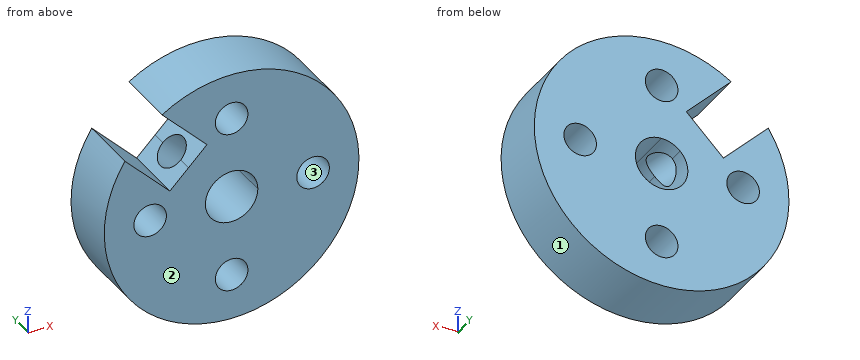
```python
from build123d import *

# Parameters (mm, degrees)
SKETCH_1_R          = 12.5
EXTRUDE_1_DEPTH     = 6
SKETCH_4_R          = 1.6
CUT_EXTRUDE_2_DEPTH = 30
CUT_EXTRUDE_3_DEPTH = 30
SKETCH_6_R          = 1.6
CUT_EXTRUDE_4_DEPTH = 6


with BuildPart() as part:
    # 草图1 → 凸台-拉伸1 (new body)
    with BuildSketch(Plane(origin=(0, 0, 0), x_dir=(1, 0, 0), z_dir=(0, 1, 0))):
        with Locations(Location((0, 0, 0), (0, 0, 270))):
            Circle(SKETCH_1_R)
    extrude(amount=EXTRUDE_1_DEPTH)

    # 草图4 → 切除-拉伸2 (cut)
    with BuildSketch(Plane(origin=(0, 0, 0), x_dir=(1, 0, 0), z_dir=(0, 1, 0))):
        with Locations(Location((0, 8, 0), (0, 0, 270))):
            Circle(SKETCH_4_R)
        with Locations(Location((8, 0, 0), (0, 0, 270))):
            Circle(SKETCH_4_R)
        with Locations(Location((0, -8, 0), (0, 0, 270))):
            Circle(SKETCH_4_R)
        with Locations(Location((-8, 0, 0), (0, 0, 270))):
            Circle(SKETCH_4_R)
    extrude(amount=CUT_EXTRUDE_2_DEPTH, mode=Mode.SUBTRACT)

    # 草图5 → 切除-拉伸3 (cut)
    with BuildSketch(Plane.XZ):
        with BuildLine():
            Line((-4.242640687, 4.242640687), (-8.838834765, 8.838834765))
            ThreePointArc((-8.838834765, 8.838834765), (-9.706634329, 7.875992001), (-10.470059323, 6.8284594))
            Line((-10.470059323, 6.8284594), (-6.063440649, 2.421840726))
            Line((-6.063440649, 2.421840726), (-4.242640687, 4.242640687))
        make_face()
        with BuildLine():
            ThreePointArc((-6.8284594, 10.470059323), (-7.875992001, 9.706634329), (-8.838834765, 8.838834765))
            Line((-8.838834765, 8.838834765), (-4.242640687, 4.242640687))
            Line((-4.242640687, 4.242640687), (-2.421840726, 6.063440649))
            Line((-2.421840726, 6.063440649), (-6.8284594, 10.470059323))
        make_face()
        with BuildLine():
            ThreePointArc((0, 2.575), (-0.985409838, 2.378989796), (-1.820799962, 1.820799962))
            Line((-1.820799962, 1.820799962), (0, 0))
            Line((0, 0), (0, 2.575))
        make_face()
        with BuildLine():
            Line((0, 0), (-1.820799962, 1.820799962))
            ThreePointArc((-1.820799962, 1.820799962), (-0.985409838, -2.378989796), (2.575, 0))
            ThreePointArc((2.575, 0), (1.820799962, 1.820799962), (0, 2.575))
            Line((0, 2.575), (0, 0))
        make_face()
    extrude(amount=-CUT_EXTRUDE_3_DEPTH, mode=Mode.SUBTRACT)

    # 草图6 → 切除-拉伸4 (cut)
    with BuildSketch(Plane(origin=(-4.242640687, 0, 4.242640687), x_dir=(0.7071067811865509, 0, 0.7071067811865442), z_dir=(-0.7071067811865442, 0, 0.7071067811865509))):
        with Locations((0, 3)):
            Circle(SKETCH_6_R)
    extrude(amount=-CUT_EXTRUDE_4_DEPTH, mode=Mode.SUBTRACT)


solid = part.part
```
Verification items for the finished model (mm, model axes). Face numbers are marked on the shaded views. Coordinates: 2 decimals unless noted, no trailing zeros. Loops run counter-clockwise (first coordinate to the right, second up) from the corner with the lowest first, then second, coordinate; pieces in that order, holes last. Notation, with made-up numbers: (83.5, 22.5) -> (119.5, 22.5) arc R20 ccw to (119.5, 33.5) -> close; hole circle Ø2 at (-10, -4.75). An arc over 180 degrees is marked (long way). Put each result on its own line as item: value.
1. Mould release check, pull along Z, two halves, no side actions. Record for the marked faces 1, 2 and 3: pulls with the +Z half, pulls with the -Z half, needs draft (parallel to the pull), parting line crosses it, or undercut.
Result set:
face 1: parting line crosses it
face 2: needs draft
face 3: undercut
2. Section check C-C, the plane y = 5.25. Record the boundary of the cut face in (x, z) (3 decimals).
Result set:
outline: (-10.47, 6.828) arc R12.5 ccw (long way) to (-6.828, 10.47) -> (-2.422, 6.063) -> (-6.063, 2.422) -> close; hole circle Ø3.2 at (-8, 0); hole circle Ø5.15 at (0, 0); hole circle Ø3.2 at (0, -8); hole circle Ø3.2 at (0, 8); hole circle Ø3.2 at (8, 0)
3. Gauge pin test, flat ends, axial feed: P1, Ø3, axis at x = 8, z = 0, coming from the +Y side; P2, Ø1.5, axis at y = 2, z = 3.5, coming from the +X side. Record the tip position at first contact, or that the pin passes through.
Result set:
P1: passes through
P2: stops at x = 12.19
4. Thickness scan on line 1 (X direction, y = 3.9, z = 0) (3 decimals); line 2 (Z direction, x = 1.25, y = 5.25). Record the ranges inside material, lowest first.
Result set:
line 1: x = -12.5 to -9.6, -6.4 to -2.575, 2.575 to 6.4, 9.6 to 12.5
line 2: z = -12.44 to -9, -7 to -2.25, 2.25 to 7, 9 to 12.44
5. Section check B-B, the plane z = -9. Record the boundary of the cut face in (x, y), then the cut area to 3 significant figures.
Result set:
outline: (-8.67, 0) -> (-1.25, 0) -> (-1.25, 6) -> (-8.67, 6) -> close; (1.25, 0) -> (8.67, 0) -> (8.67, 6) -> (1.25, 6) -> close
area: 89.1 mm^2
6. Section check D-D, the plane z = 3. Give the number of separate pieces and of enclosed holes in the cut face, then the cut area to 3 significant figures.
Result set:
separate pieces: 2
enclosed holes: 1
area: 127 mm^2
7. Section check A-A, the plane x = -8. Record the boundary of the cut face in (y, z).
Result set:
outline: (0, -9.6) -> (6, -9.6) -> (6, -1.6) -> (0, -1.6) -> close; (0, 1.6) -> (6, 1.6) -> (6, 4.36) -> (0, 4.36) -> close
